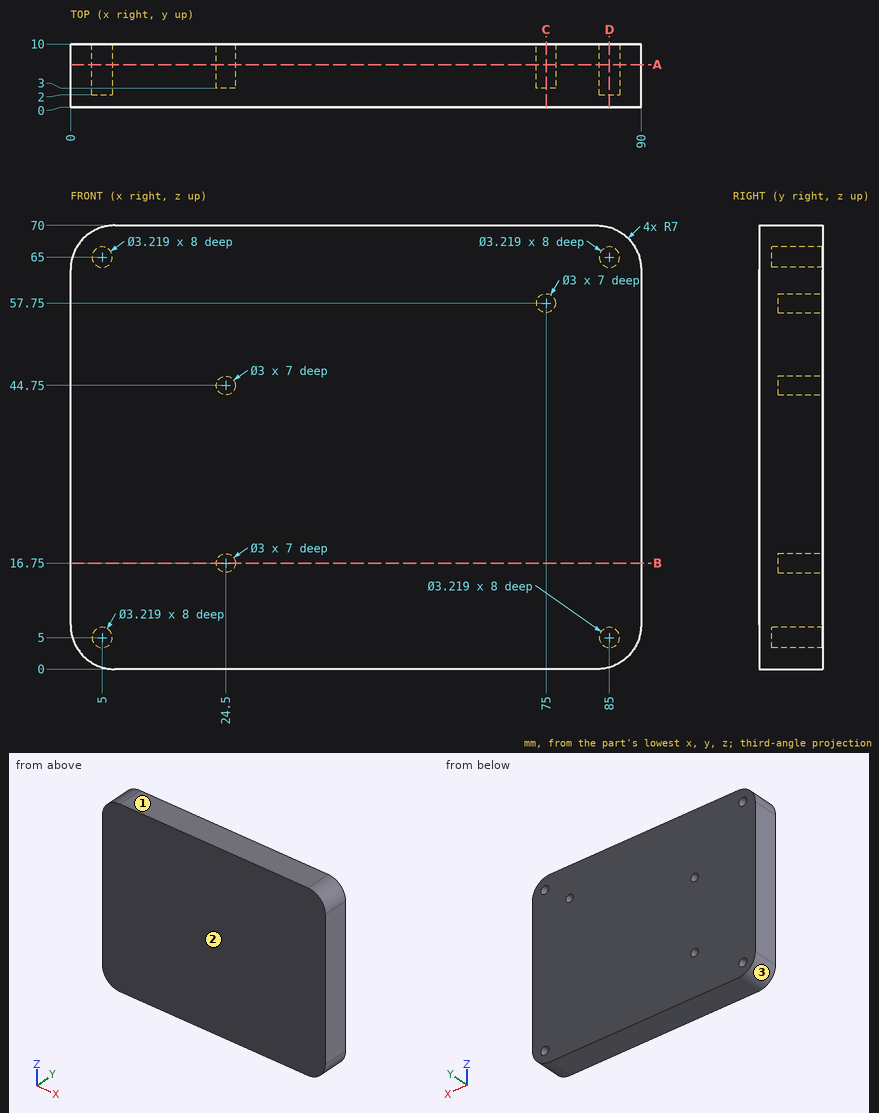
Check sheet for the drawn part. Datum: minimum x, y, z corner. Units: mm. Coordinates: 2 decimals unless noted, no trailing zeros. Order: outer loops, then holes, each group sorted by start corner. A loop starts at its lowest first (then second) coordinate and runs counter-clockwise, first axis right, second up. Notation, with made-up numbers: (85, 7) -> (121, 7) arc R26 cw to (121, 30) -> close; hole circle Ø9 at (58.5, 44). An arc over 180 degrees is marked (long way). Use a Markdown table: item, result. Add a question column.
1. Cross-section at B-B (z = 16.75). Enter the section's corners in (x, y).
2. Go/stop test with flat-tipped pins: pin 1 Ø0.9 at (x, z) = (74.5, 57.5) entering from +Y; pin 2 Ø1.9 at (x, z) = (5, 65) entering from +Y. Record where each tip stops, or that it passes through.
3. Mould release check, pull along Z, two halves, no side actions. Record for the marked faces 1, 2 and 3: pulls with the +Z half, pulls with the -Z half, needs draft (parallel to the pull), parting line crosses it, or undercut.
4. Cross-section at D-D (x = 85). Enter the section's corners in (y, z), and give its area (3 significant figures).
5. Material ranges on L1, parallel to Z at x = 24.5, y = 5.5; L2, parallel to X at y = 5, z = 44.75; L3, parallel to X at y = 6.75, z = 5, recorded low to high.
6. Cross-section at C-C (x = 75). Enter the section's corners in (y, z), and give its area (3 significant figures).
7. Cross-section at A-A (y = 6.75). Enter the section's corners in (x, z), and give its area (3 significant figures).
Filled sheet:
| question | item | result |
|---|---|---|
| 1 | outline | (0, 0) -> (90, 0) -> (90, 10) -> (26, 10) -> (26, 3) -> (23, 3) -> (23, 10) -> (0, 10) -> close |
| 2 | pin 1 | y = 3 |
| 2 | pin 2 | y = 2 |
| 3 | face 1 | pulls with the +Z half |
| 3 | face 2 | needs draft |
| 3 | face 3 | pulls with the -Z half |
| 4 | outline | (0, 0.29) -> (10, 0.29) -> (10, 3.39) -> (2, 3.39) -> (2, 6.61) -> (10, 6.61) -> (10, 63.39) -> (2, 63.39) -> (2, 66.61) -> (10, 66.61) -> (10, 69.71) -> (0, 69.71) -> close |
| 4 | area | 643 mm2 |
| 5 | L1 | 0 to 15.25, 18.25 to 43.25, 46.25 to 70 |
| 5 | L2 | 0 to 23, 26 to 90 |
| 5 | L3 | 0.29 to 3.39, 6.61 to 83.39, 86.61 to 89.71 |
| 6 | outline | (0, 0) -> (10, 0) -> (10, 56.25) -> (3, 56.25) -> (3, 59.25) -> (10, 59.25) -> (10, 70) -> (0, 70) -> close |
| 6 | area | 679 mm2 |
| 7 | outline | (0, 7) arc R7 ccw to (7, 0) -> (83, 0) arc R7 ccw to (90, 7) -> (90, 63) arc R7 ccw to (83, 70) -> (7, 70) arc R7 ccw to (0, 63) -> close; hole circle Ø3.22 at (5, 5); hole circle Ø3.22 at (5, 65); hole circle Ø3 at (24.5, 16.75); hole circle Ø3 at (24.5, 44.75); hole circle Ø3 at (75, 57.75); hole circle Ø3.22 at (85, 5); hole circle Ø3.22 at (85, 65) |
| 7 | area | 6,200 mm2 |
